The listing builds one solid part. Answer for the finished solid, in the listing's coordinates (mm). A direction names the side the tool comes from. Coordinates: 2 decimals unless noted, no trailing zeros. Order: outer loops, then holes, each group sorted by start corner. A loop starts at its lowest first (then second) coordinate and runs counter-clockwise, first axis right, second up.
Autodesk Inventor part; units mm, degrees
ref_plane "YZ Plane" through (0, 0, 0) normal (1, 0, 0) x (0, 1, 0)
ref_plane "XZ Plane" through (0, 0, 0) normal (0, 1, 0) x (-1, 0, 0)
ref_plane "XY Plane" through (0, 0, 0) normal (0, 0, 1) x (1, 0, 0)
sketch "Sketch1" plane through (0, 0, 0) normal (0, 0, 1) x (1, 0, 0)
  circle A0 centre (0, 0) radius 1.65
  circle A1 centre (0, 0) radius 1.35
  point P0 (0, 0)
  dimension "d21" = 2.7
extrude "Extrusion1" add sketch "Sketch1" along normal blind 5 and the other way blind 15 contours A1
sketch "Sketch2" plane through (0, 0, 5) normal (0, 0, 1) x (1, 0, 0)
  circle A0 centre (0, 0) radius 1.35
  line L0 (-0.9546, 0.9546) -> (0.9546, 0.9546)
  line L1 (0.9546, 0.9546) -> (0.9546, -0.9546)
  line L2 (0.9546, -0.9546) -> (-0.9546, -0.9546)
  line L3 (-0.9546, -0.9546) -> (-0.9546, 0.9546)
  circle A1 centre (0, 0) radius 1.35
  point P0 (0, 0)
extrude "Extrusion2" cut sketch "Sketch2" against normal blind 2 contours A0 L1 | L0 A0 | A0 L2 | L3 A0
sketch "Sketch3" plane through (0, 0, 3) normal (0, 0, 1) x (1, 0, 0)
  arc A0 (-0.9546, 0.9546) -> (-0.9546, -0.9546) centre (0, 0) ccw
  arc A1 (0.9546, 0.9546) -> (-0.9546, 0.9546) centre (0, 0) ccw
  arc A2 (0.9546, -0.9546) -> (0.9546, 0.9546) centre (0, 0) ccw
  arc A3 (-0.9546, -0.9546) -> (0.9546, -0.9546) centre (0, 0) ccw
  arc A4 (-0.9546, 0.9546) -> (-0.9546, -0.9546) centre (0, 0) ccw
  circle A5 centre (0, 0) radius 1.35
  circle A6 centre (0, 0) radius 1.9092
  point P0 (0, 0)
extrude "Extrusion3" add sketch "Sketch3" against normal blind 2.7
sketch "Sketch4" plane through (0, 0, -15) normal (0, 0, -1) x (-1, 0, 0)
  circle A0 centre (0, 0) radius 1.35
  circle A1 centre (0, 0) radius 1.35
  circle A2 centre (0, 0) radius 1.9092
  line L0 (-0.9546, -0.9546) -> (-0.9546, 0.9546)
  line L1 (0.9546, -0.9546) -> (-0.9546, -0.9546)
  line L2 (0.9546, 0.9546) -> (0.9546, -0.9546)
  line L3 (-0.9546, 0.9546) -> (0.9546, 0.9546)
extrude "Extrusion4" cut sketch "Sketch4" against normal blind 2 contours A0 L2 | L3 A0 | A0 L1 | L0 A0
sketch "Sketch5" plane through (0, 0, -13) normal (0, 0, -1) x (-1, 0, 0)
  circle A0 centre (0, 0) radius 1.9092
  point P0 (0, 0)
extrude "Extrusion5" add sketch "Sketch5" against normal blind 2.7
sketch "Sketch7" plane through (-0.9546, -0.9546, -15) normal (0, -1, 0) x (1, 0, 0)
  line L0 (1.9092, 2) -> (0, 2) construction
  line L1 (0, 0) -> (0, 2) construction
  line L2 (1.9092, 2) -> (1.9092, 0) construction
  line L3 (-1.4999, 2) -> (3.4091, 2)
  line L4 (3.4091, 2) -> (3.4091, 0)
  line L5 (3.4091, 0) -> (-1.4999, 0)
  line L6 (-1.4999, 0) -> (-1.4999, 2)
  line L7 (0.9546, 19.9961) -> (0.9546, 0)
  line L8 (0.9546, 9.998) -> (8.9961, 9.998)
  line L9 (-1.4999, 17.9961) -> (3.4091, 17.9961)
  line L10 (3.4091, 17.9961) -> (3.4091, 19.9961)
  line L11 (3.4091, 19.9961) -> (-1.4999, 19.9961)
  line L12 (-1.4999, 19.9961) -> (-1.4999, 17.9961)
  point P0 (0.9546, 15)
  dimension "d13" = 4.909
  dimension "d14" = 1.4999
  dimension "d15" = 1.9092
  dimension "d16" = 2
  dimension "d17" = 2
  dimension "d18" = 0
extrude "Extrusion6" add sketch "Sketch7" against normal up to surface (1.9092 mm away)
sketch "Sketch8" plane through (0, 0, -10.3) normal (0, 0, 1) x (1, 0, 0)
  circle A0 centre (0, 0) radius 1.35
  circle A1 centre (0, 0) radius 3.375
  dimension "d22" = 2.7
  dimension "d23" = 6.75
extrude "Extrusion7" add sketch "Sketch8" along normal up to surface (10.6 mm away)
sketch "Sketch9" plane through (0, 0, -10.3) normal (0, 0, -1) x (-1, 0, 0)
  circle A0 centre (0, 0) radius 3.375
  circle A1 centre (0, 0) radius 1.9092
  circle A2 centre (0, 0) radius 4.375
  dimension "d26" = 1
extrude "Extrusion8" add sketch "Sketch9" along normal up to surface (2.7 mm away) contours A0 | A2
sketch "Sketch10" plane through (0, 0, 0.3) normal (0, 0, 1) x (1, 0, 0)
  circle A0 centre (0, 0) radius 1.9092
  circle A1 centre (0, 0) radius 4.375
extrude "Extrusion9" add sketch "Sketch10" along normal up to surface (2.7 mm away)
sketch "Sketch12" plane through (0, 0, 3) normal (0, 0, 1) x (1, 0, 0)
  circle A0 centre (0, 0) radius 4.375
  line L0 (2.4545, -0.9546) -> (-2.4545, -0.9546)
  line L1 (-2.4545, 0.9546) -> (-2.4545, -0.9546)
  line L2 (2.4545, 0.9546) -> (-2.4545, 0.9546)
  line L3 (2.4545, -0.9546) -> (2.4545, 0.9546)
extrude "Extrusion11" cut sketch "Sketch12" against normal blind 0.3
sketch "Sketch13" plane through (0, 0, -13) normal (0, 0, -1) x (-1, 0, 0)
  circle A0 centre (0, 0) radius 4.375
  line L0 (-2.4545, 0.9546) -> (2.4545, 0.9546)
  line L1 (2.4545, -0.9546) -> (2.4545, 0.9546)
  line L2 (-2.4545, -0.9546) -> (2.4545, -0.9546)
  line L3 (-2.4545, -0.9546) -> (-2.4545, 0.9546)
extrude "Extrusion12" cut sketch "Sketch13" against normal blind 0.3
sketch "Sketch14" plane through (0, 0, -10.3) normal (0, 0, 1) x (1, 0, 0)
  circle A0 centre (0, 0) radius 3.375
  circle A1 centre (0, 0) radius 4.1
  dimension "d37" = 8.2
extrude "Extrusion13" add sketch "Sketch14" along normal up to surface (10.6 mm away)
sketch "Sketch15" plane through (0, 0, -12.7) normal (0, 0, -1) x (-1, 0, 0)
  circle A0 centre (0, 0) radius 4.375
  line L0 (-4.375, 4.375) -> (4.375, 4.375)
  line L1 (4.375, 4.375) -> (4.375, -4.375)
  line L2 (4.375, -4.375) -> (-4.375, -4.375)
  line L3 (-4.375, -4.375) -> (-4.375, 4.375)
  dimension "d40" = 8.75
  dimension "d41" = 8.75
  dimension "d42" = 8.75
extrude "Extrusion14" add sketch "Sketch15" against normal up to surface (2.4 mm away) contours L1 L2 A0 | A0 L0 L1 | A0 L3 L0 | L2 L3 A0
sketch "Sketch16" plane through (0, 0, 2.7) normal (0, 0, 1) x (1, 0, 0)
  circle A0 centre (0, 0) radius 4.375
  line L0 (2.4545, 0.9546) -> (2.4545, -0.9546)
  line L1 (-2.4545, 0.9546) -> (2.4545, 0.9546)
  line L2 (-2.4545, -0.9546) -> (-2.4545, 0.9546)
  line L3 (2.4545, -0.9546) -> (-2.4545, -0.9546)
  line L4 (-4.375, 4.375) -> (-4.375, -4.375)
  line L5 (4.375, 4.375) -> (-4.375, 4.375)
  line L6 (4.375, -4.375) -> (4.375, 4.375)
  line L7 (-4.375, -4.375) -> (4.375, -4.375)
extrude "Extrusion15" add sketch "Sketch16" against normal up to surface (2.4 mm away) contours L6 L7 A0 | A0 L5 L6 | A0 L4 L5 | L7 L4 A0
sketch "Sketch17" plane through (0, 0, 2.7) normal (0, 0, 1) x (1, 0, 0)
  line L0 (2.4545, -0.9546) -> (2.4545, 0.9546)
  line L1 (-2.4545, -0.9546) -> (2.4545, -0.9546)
  line L2 (-2.4545, 0.9546) -> (-2.4545, -0.9546)
  line L3 (2.4545, 0.9546) -> (-2.4545, 0.9546)
  line L4 (-4.375, 4.375) -> (4.375, 4.375)
  line L5 (-4.375, -4.375) -> (-4.375, 4.375)
  line L6 (4.375, -4.375) -> (-4.375, -4.375)
  line L7 (4.375, 4.375) -> (4.375, -4.375)
  point P0 (0, 0)
extrude "Extrusion16" add sketch "Sketch17" along normal up to surface (2.2961 mm away)
sketch "Sketch18" plane through (0, 0, -12.7) normal (0, 0, -1) x (-1, 0, 0)
  line L0 (-2.4545, 0.9546) -> (-2.4545, -0.9546)
  line L1 (2.4545, 0.9546) -> (-2.4545, 0.9546)
  line L2 (2.4545, -0.9546) -> (2.4545, 0.9546)
  line L3 (-2.4545, -0.9546) -> (2.4545, -0.9546)
  line L4 (4.375, 4.375) -> (4.375, -4.375)
  line L5 (-4.375, 4.375) -> (4.375, 4.375)
  line L6 (-4.375, -4.375) -> (-4.375, 4.375)
  line L7 (4.375, -4.375) -> (-4.375, -4.375)
  point P0 (0, 0)
extrude "Extrusion17" add sketch "Sketch18" along normal up to surface (2.3 mm away)
sketch "Sketch19" plane through (0, 0, 0.3) normal (0, 0, -1) x (-1, 0, 0)
  circle A0 centre (0, 0) radius 4.1
  circle A1 centre (0, 0) radius 2.6
  dimension "d51" = 1.5
extrude "Extrusion18" cut sketch "Sketch19" along normal up to surface (10.6 mm away) contours A1
equation "\"d14\" = -0.5 * d15 + 0.5 * d13"
equation "\"d23\" = 2.5 * d22"
equation "\"d41\" = d40"
equation "\"d42\" = d40"
properties part number "LargeSmallGearAxis"
1) A cutting plane is placed at D-D, the plane x = -2. Write down the section's boundary in (y, z) (3 decimals).
2) Each of these flat-tipped pins is pushed along its axis until it touches: P1, Ø1.5, axis at x = -2, z = -1, coming from the +Y side; P2, Ø3, axis at x = -1, y = 3.5, coming from the +Z side. Where does it stop, or does it pass through?
3) A cutting plane is placed at C-C, the plane z = -1.75. Write down the section's boundary in (x, y).
4) For faces 4 (the flat face through (-4.375, 0, 3)), 5 (the flat face through (4, 2, -10.3)), determine the directions among +Z, -Z, +X, -X, +Y, -Y from which every point of the face is accessible in a straight line to the end or side of a thin tool.
5) Straight lines are drawn through the part: probe 1 along Z at (x, y) = (-3, 3.25); probe 2 along Y at (x, z) = (0, -6.5); probe 3 along Z at (x, y) = (3, 0.75). For each, find the intervals that lie inside material, in ascending order.
6) The mould has two halves that part along Z. Classify faces 1 (the flat face through (0, 2, 4.996)), 2 (the cylindrical face through (0.338, -2.578, -4.926)), 3 (the flat face through (0, 4.375, 3)): released by +Z, released by -Z, zero draft, split by the parting line, or undercut.
Working result:
1. outline: (-4.375, -15) - (4.375, -15) - (4.375, -10.3) - (3.579, -10.3) - (3.579, 0.3) - (4.375, 0.3) - (4.375, 4.996) - (-4.375, 4.996) - (-4.375, 0.3) - (-3.579, 0.3) - (-3.579, -10.3) - (-4.375, -10.3) - close; hole (-1.661, -10.3) - (1.661, -10.3) - (1.661, 0.3) - (-1.661, 0.3) - close
2. P1: stops at y = 3.9
2. P2: stops at z = 5
3. outline: circle Ø8.2 at (0, 0); hole circle Ø5.2 at (0, 0)
4. face 4: +Z, -Z, -X, +Y, -Y
4. face 5: none
5. probe 1: z = -15 to -10.3, 0.3 to 5
5. probe 2: y = -4.1 to -2.6, 2.6 to 4.1
5. probe 3: z = -15 to 5
6. face 1: released by +Z
6. face 2: undercut
6. face 3: zero draft
